```python
from build123d import *

# Parameters (mm, degrees)
ESBO_O1_R                = 1.599999999999999
ESBO_O1_R_2              = 1.600000000000006
ESBO_O1_R_3              = 1.5999999999999974
ESBO_O1_R_4              = 1.5999999999999985
ESBO_O1_R_5              = 1.5999999999999979
ESBO_O1_R_6              = 1.600000000000005
ESBO_O1_R_7              = 3.0000000000000013
RESSALTO_EXTRUS_O1_DEPTH = 6
FILETE1_R                = 10
FILETE2_R                = 5
FILETE4_R                = 5
FILETE5_R                = 3
CHANFRO1_SIZE            = 15
CHANFRO1_SIZE2           = 10.50311307314568
FILETE6_R                = 5


# Some blends are built 0.0001 mm under size
with BuildPart() as part:
    # Esboço1 → Ressalto-extrusão1 (new body)
    with BuildSketch(Plane.XY):
        Polygon((10.000000000000002, -2e-17), (9.999999999999998, 30.00000000000003), (-10.000000000000002, 30.000000000000025), (-10.000000000000002, 23.000000000000007), (-15.00000000000002, 22.99999999999999), (-15, 16.999999999999996), (-25, 17), (-25.000000000000007, 22.999999999999993), (-66.7010377283415, 23.00000000000001), (-80.7428791412217, -37.388961654722294), (-65.64563872754113, -40.899422007942356), (-66.49494365170727, -44.55198017254248), (-56.754788546106894, -46.81679330365219), (-55.90548362194075, -43.16423513905207), (-40.8082432082602, -46.674695492272136), (-29.95528839436153, 0), (-5.0000000000000036, -3e-17), (-5.000000000000001, 5.999999999999998), (4.999999999999999, 6), (5, -9.54e-15), align=None)
        with Locations((-60.49245953335221, -40.814309185297155)):
            Circle(ESBO_O1_R, mode=Mode.SUBTRACT)
        with Locations((-64.23013052059758, -34.81182506694214)):
            Circle(ESBO_O1_R_2, mode=Mode.SUBTRACT)
        with Locations((-54.48997541499719, -37.07663819805185)):
            Circle(ESBO_O1_R_3, mode=Mode.SUBTRACT)
        Polygon((-70.14267850253108, -18.293523811627352), (-73.06472503421121, -17.614079872294436), (-68.53509877199178, 1.8662303389063057), (-65.61305224031166, 1.1867863995733938), align=None, mode=Mode.SUBTRACT)
        Polygon((-48.28358518275084, -34.66972725556205), (-68.73791090451164, -29.91361968023165), (-59.22569575385083, 10.995031763289926), (-38.771370032090054, 6.238924187959523), align=None, mode=Mode.SUBTRACT)
        Polygon((-34.44455590239049, -6.060615619977673), (-38.97418216460991, -25.540925831178406), (-41.89622869629001, -24.861481891845497), (-37.3666024340706, -5.3811716806447585), align=None, mode=Mode.SUBTRACT)
        with Locations((-60.67691042150691, 18.000000000000004)):
            Circle(ESBO_O1_R_4, mode=Mode.SUBTRACT)
        with Locations((-53.019305521604494, 13.40194270577972)):
            Circle(ESBO_O1_R_5, mode=Mode.SUBTRACT)
        with Locations((-43.2791504160041, 11.137129574670004)):
            Circle(ESBO_O1_R_6, mode=Mode.SUBTRACT)
        with Locations((-2.44e-15, 20)):
            Circle(ESBO_O1_R_7, mode=Mode.SUBTRACT)
    extrude(amount=RESSALTO_EXTRUS_O1_DEPTH)

    # Filete1
    filete1_edges = [part.edges().sort_by_distance(p)[0] for p in [
        (-29.95528839436153, -3e-17, 3),
    ]]
    fillet(filete1_edges, radius=FILETE1_R)

    # Filete2
    # the kernel refuses this fillet: 5 mm, written as the material it takes off along each edge
    with BuildSketch(Plane(origin=(-66.70103772834149, 23.00000000000001, -9.926929788370014), x_dir=(-0.22648131311097233, -0.974015510560037, 0), z_dir=(0, 0, 1))) as filete2_piece_1:
        with BuildLine():
            CenterArc((FILETE2_R * 0.79415438307, FILETE2_R), FILETE2_R, 193.08999999999958, 76.91000000000048)
            Line((-FILETE2_R * 0.17986112749, FILETE2_R * 0.773518686889), (-FILETE2_R * 0.199341437702, FILETE2_R * 0.768989060627))
            Line((-FILETE2_R * 0.199341437702, FILETE2_R * 0.768989060627), (-FILETE2_R * 0.0158830876614, -FILETE2_R * 0.02))
            Line((-FILETE2_R * 0.0158830876614, -FILETE2_R * 0.02), (FILETE2_R * 0.79415438307, -FILETE2_R * 0.02))
            Line((FILETE2_R * 0.79415438307, -FILETE2_R * 0.02), (FILETE2_R * 0.79415438307, 6e-17))
        make_face()
    extrude(amount=25.853859576740028, mode=Mode.SUBTRACT)
    with BuildSketch(Plane(origin=(-66.49494365170727, -44.55198017254248, -12.103072956898195), x_dir=(0.9740155105600374, -0.22648131311097125, 0), z_dir=(0, 0, 1))) as filete2_piece_2:
        with BuildLine():
            CenterArc((4.841229182759275, 5.000000000000003), FILETE2_R, 194.4775121859302, 75.52248781406985)
            Line((1.133e-14, 3.7499999999999782), (-0.09682458365516827, 3.7249999999999814))
            ThreePointArc((-0.09682458365516827, 3.7249999999999814), (-0.10000000000000146, 1.874999999999995), (-0.10000000000000632, 2.39e-15))
            Line((-0.10000000000000632, 2.39e-15), (-4e-15, -0.0999999999999994))
            Line((-4e-15, -0.0999999999999994), (4.841229182759282, -0.09999999999999787))
            Line((4.841229182759282, -0.09999999999999787), (4.841229182759279, -9e-17))
        make_face()
    extrude(amount=30.20614591379639, mode=Mode.SUBTRACT)
    with BuildSketch(Plane(origin=(-56.754788546106894, -46.81679330365219, -12.103072956898142), x_dir=(0.22648131311097194, 0.9740155105600371, 0), z_dir=(0, 0, 1))) as filete2_piece_3:
        with BuildLine():
            CenterArc((4.9999999999999964, 4.841229182759264), FILETE2_R, 180.00000000000009, 75.52248781406979)
            Line((-5.64e-15, 4.841229182759256), (-0.10000000000000338, 4.841229182759253))
            Line((-0.10000000000000338, 4.841229182759253), (-0.09999999999999777, -2.99e-15))
            Line((-0.09999999999999777, -2.99e-15), (2.99e-15, -0.09999999999999777))
            ThreePointArc((2.99e-15, -0.09999999999999777), (1.8749999999999951, -0.10000000000000121), (3.724999999999985, -0.09682458365518365))
            Line((3.724999999999985, -0.09682458365518365), (3.7499999999999827, 3e-17))
        make_face()
    extrude(amount=30.206145913796284, mode=Mode.SUBTRACT)
    with BuildSketch(Plane(origin=(-40.8082432082602, -46.674695492272136, -12.500000000000021), x_dir=(0.22648131311097006, 0.9740155105600377, 0), z_dir=(0, 0, 1))) as filete2_piece_4:
        with BuildLine():
            CenterArc((FILETE2_R, FILETE2_R), FILETE2_R, 179.9999999999999, 90)
            Line((2.239e-14, FILETE2_R), (-FILETE2_R * 0.02, FILETE2_R))
            Line((-FILETE2_R * 0.02, FILETE2_R), (-FILETE2_R * 0.02, -FILETE2_R * 0.02))
            Line((-FILETE2_R * 0.02, -FILETE2_R * 0.02), (FILETE2_R, -FILETE2_R * 0.02))
            Line((FILETE2_R, -FILETE2_R * 0.02), (FILETE2_R, 6e-17))
        make_face()
    extrude(amount=31.000000000000043, mode=Mode.SUBTRACT)
    with BuildSketch(Plane(origin=(-10.000000000000002, 30.000000000000025, -12.499999999999996), x_dir=(1, 0, 0), z_dir=(0, 0, 1))) as filete2_piece_5:
        with BuildLine():
            CenterArc((FILETE2_R, -FILETE2_R), FILETE2_R, 90.00000000000001, 89.99999999999996)
            Line((-1.78e-15, -FILETE2_R), (-FILETE2_R * 0.02, -FILETE2_R))
            Line((-FILETE2_R * 0.02, -FILETE2_R), (-FILETE2_R * 0.02, FILETE2_R * 0.02))
            Line((-FILETE2_R * 0.02, FILETE2_R * 0.02), (FILETE2_R, FILETE2_R * 0.02))
            Line((FILETE2_R, FILETE2_R * 0.02), (FILETE2_R, 0))
        make_face()
    extrude(amount=30.999999999999993, mode=Mode.SUBTRACT)
    with BuildSketch(Plane(origin=(9.999999999999998, 30.00000000000003, -12.5), x_dir=(0, -1, 0), z_dir=(0, 0, 1))) as filete2_piece_6:
        with BuildLine():
            CenterArc((FILETE2_R, -FILETE2_R), FILETE2_R, 90, 90)
            Line((0, -FILETE2_R), (-FILETE2_R * 0.02, -FILETE2_R))
            Line((-FILETE2_R * 0.02, -FILETE2_R), (-FILETE2_R * 0.02, FILETE2_R * 0.02))
            Line((-FILETE2_R * 0.02, FILETE2_R * 0.02), (FILETE2_R, FILETE2_R * 0.02))
            Line((FILETE2_R, FILETE2_R * 0.02), (FILETE2_R, 0))
        make_face()
    extrude(amount=31, mode=Mode.SUBTRACT)

    # Filete4
    filete4_edges = [part.edges().sort_by_distance(p)[0] for p in [
        (-65.64563872754113, -40.89942200794236, 3),
        (-55.90548362194075, -43.16423513905207, 3),
        (-10.000000000000002, 23, 3),
    ]]
    fillet(filete4_edges, radius=FILETE4_R - 0.0001)  # a hair under: the kernel refuses the full size

    # Filete5
    # the kernel refuses this fillet: 3 mm, written as the material it takes off along each edge
    with BuildSketch(Plane(origin=(-25.000000000000007, 23.000000000000007, -7.499999999999991), x_dir=(-1, 0, 0), z_dir=(0, 0, 1))) as filete5_piece_1:
        with BuildLine():
            CenterArc((FILETE5_R, FILETE5_R), FILETE5_R, 180.00000000000006, 89.99999999999994)
            Line((-3.55e-15, FILETE5_R), (0, 0))
            Line((0, 0), (FILETE5_R, 0))
        make_face()
    extrude(amount=20.99999999999998, mode=Mode.SUBTRACT)
    with BuildSketch(Plane(origin=(-15.00000000000002, 22.99999999999999, -6.465722061975505), x_dir=(3.43e-15, -1, 0), z_dir=(0, 0, 1))) as filete5_piece_2:
        with BuildLine():
            CenterArc((2.5862888247905, 3), FILETE5_R, 198.50689627931516, 71.49310372068487)
            Line((-0.25856754520870956, 2.0477436090658623), (-0.5430531822086313, 1.9525179699724493))
            ThreePointArc((-0.5430531822086313, 1.9525179699724493), (-0.2999999999996936, 0.4606813660513637), (-0.3000000000000007, 1.03e-15))
            Line((-0.3000000000000007, 1.03e-15), (-1.03e-15, -0.3000000000000007))
            Line((-1.03e-15, -0.3000000000000007), (2.5862888247904996, -0.3000000000000007))
            Line((2.5862888247904996, -0.3000000000000007), (2.5862888247905005, 0))
        make_face()
    extrude(amount=18.93144412395101, mode=Mode.SUBTRACT)
    with BuildSketch(Plane(origin=(-5.0000000000000036, -3e-17, -7.5), x_dir=(-1, 1e-17, 0), z_dir=(0, 0, 1))) as filete5_piece_3:
        with BuildLine():
            CenterArc((FILETE5_R, -FILETE5_R), FILETE5_R, 90, 90)
            Line((3e-17, -FILETE5_R), (0, 0))
            Line((0, 0), (FILETE5_R, 0))
        make_face()
    extrude(amount=21, mode=Mode.SUBTRACT)
    with BuildSketch(Plane(origin=(10.000000000000002, -2e-17, -7.500000000000002), x_dir=(-1, 1e-17, 0), z_dir=(0, 0, 1))) as filete5_piece_4:
        with BuildLine():
            CenterArc((FILETE5_R, -FILETE5_R), FILETE5_R, 90, 90)
            Line((1.79e-15, -FILETE5_R), (0, 0))
            Line((0, 0), (FILETE5_R, 0))
        make_face()
    extrude(amount=21, mode=Mode.SUBTRACT)
    with BuildSketch(Plane(origin=(5, 0, -7.5), x_dir=(-3e-16, 1, 0), z_dir=(0, 0, 1))) as filete5_piece_5:
        with BuildLine():
            CenterArc((FILETE5_R, -FILETE5_R), FILETE5_R, 90, 90)
            Line((-8.9e-16, -FILETE5_R), (0, 0))
            Line((0, 0), (FILETE5_R, 0))
        make_face()
    extrude(amount=21, mode=Mode.SUBTRACT)

    # Chanfro1
    chanfro1_edges = [part.edges().sort_by_distance(p)[0] for p in [
        (-80.7428791412217, -37.388961654722294, 3),
    ]]
    chanfro1_side = [part.faces().sort_by_distance(p)[0] for p in [
        (-74.1716112535079, -9.128277544584641, 3),
    ]]
    chamfer(chanfro1_edges, length=CHANFRO1_SIZE, length2=CHANFRO1_SIZE2, reference=chanfro1_side[0])

    # Filete6
    filete6_edges = [part.edges().sort_by_distance(p)[0] for p in [
        (-77.34565944455714, -22.778728996321732, 3),
        (-70.51268409881192, -39.76772049528134, 3),
    ]]
    fillet(filete6_edges, radius=FILETE6_R)


solid = part.part
```
Design review of the part built by this model. Coordinates are the model's own, in mm. A direction names the side the tool comes from. Coordinates: 2 decimals unless noted, no trailing zeros. Order: outer loops, then holes, each group sorted by start corner. A loop starts at its lowest first (then second) coordinate and runs counter-clockwise, first axis right, second up. Notation, with made-up numbers: (25, 77.5) - (54, 77.5) arc R19 ccw to (54, 111.5) - close; hole circle Ø1 at (-37, 20.25). An arc over 180 degrees is marked (long way). Answer in a Markdown table with one row per item.
(1) Consider section A-A on x = 0. State the section outline as (y, z) points, plus the area to 3 significant figures.
Checked values:
| item | result |
|---|---|
| outline | (6, 0) - (17, 0) - (17, 6) - (6, 6) - close; (23, 0) - (30, 0) - (30, 6) - (23, 6) - close |
| area | 108 mm^2 |
(2) Consider section B-B on x = -64. State the section outline as (y, z) points.
Checked values:
| item | result |
|---|---|
| outline | (-44.49, 0) - (-36.4, 0) - (-36.4, 6) - (-44.49, 6) - close; (-33.23, 0) - (-31.02, 0) - (-31.02, 6) - (-33.23, 6) - close; (-9.54, 0) - (22.84, 0) - (22.84, 6) - (-9.54, 6) - close |
(3) Consider section D-D on y = 7.5. State the section outline as (x, z) points, plus the area to 3 significant figures.
Checked values:
| item | result |
|---|---|
| outline | (-70.31, 0) - (-60.04, 0) - (-60.04, 6) - (-70.31, 6) - close; (-44.19, 0) - (10, 0) - (10, 6) - (-44.19, 6) - close |
| area | 387 mm^2 |
(4) The part is to be moulded in two halves that separate along X. For faces 5 (the cylindrical face through (-55.21, -43.82, 3.04)), 6 (the flat face through (-35.77, -25.01, 2.96)), 7 (the flat face through (-15, 0, 3)), say which applies: released by +X, released by -X, zero draft, split by the parting line, or undercut.
Checked values:
| item | result |
|---|---|
| face 5 | undercut |
| face 6 | released by +X |
| face 7 | zero draft |
(5) Consider section C-C on y = 18. State the section outline as (x, z) points.
Checked values:
| item | result |
|---|---|
| outline | (-67.86, 0) - (-62.28, 0) - (-62.28, 6) - (-67.86, 6) - close; (-59.08, 0) - (-25, 0) - (-25, 6) - (-59.08, 6) - close; (-15, 0) - (-2.24, 0) - (-2.24, 6) - (-15, 6) - close; (2.24, 0) - (10, 0) - (10, 6) - (2.24, 6) - close |
(6) Wall thickness on line 1 along X through (y, z) = (-24, 3.75); line 2 along Y through (x, z) = (-53.5, 2.5); line 3 along X through (y, z) = (-22, 4): over which ranges is each line inside the solid? List them lowest first. Write a range as from..to.
Checked values:
| item | result |
|---|---|
| line 1 | -76.85..-67.36, -45.8..-41.7, -38.62..-35.54 |
| line 2 | -43.75..-38.33, -35.82..-33.46, 9.66..11.88, 14.93..23 |
| line 3 | -77.1..-66.9, -45.34..-41.23, -38.15..-35.07 |
(7) For faces 1 (the flat face through (-70.83, -8.01, 2.96)), 2 (the flat face through (0, 30, 3)), 3 (the cylindrical face through (-25.86, 22.1, 2.96)), 4 (the flat face through (-5, 4, 3)), list the 3-axis set-ups (+Z, -Z, +X, -X, +Y, -Y) from which the entire face can be reached by the end or side of a thin tool; tool diameter is ignored.
Checked values:
| item | result |
|---|---|
| face 1 | +Z, -Z |
| face 2 | +Z, -Z, +X, -X, +Y |
| face 3 | +Z, -Z, +Y |
| face 4 | +Z, -Z, -Y |
(8) Clearance check with flat-ended pins moving along their axes: pin 1 (5 mm diameter, centred on x = -60.49, y = -40.81, fed in from +Z); pin 2 (2.5 mm diameter, centred on y = 19.5, z = 3, fed in from -X); pin 3 (1 mm diameter, centred on x = -22.5, z = 1, fed in from +Y); pin 4 (3.5 mm diameter, centred on x = 0, y = 20, fed in from +Z). State where each tip first meets the part, or that it passes through.
Checked values:
| item | result |
|---|---|
| pin 1 | z = 6 |
| pin 2 | x = -67.81 |
| pin 3 | y = 17 |
| pin 4 | through |
